Geometry check sheet. Reference: the model listing, model coordinates, mm. A direction names the side the tool comes from. Coordinates: 2 decimals unless noted, no trailing zeros. Order: outer loops, then holes, each group sorted by start corner. A loop starts at its lowest first (then second) coordinate and runs counter-clockwise, first axis right, second up.
Autodesk Inventor part; units mm, degrees
ref_plane "YZ Plane" through (0, 0, 0) normal (1, 0, 0) x (0, 1, 0)
ref_plane "XZ Plane" through (0, 0, 0) normal (0, 1, 0) x (-1, 0, 0)
ref_plane "XY Plane" through (0, 0, 0) normal (0, 0, 1) x (1, 0, 0)
sketch "Эскиз1" plane through (0, 0, 0) normal (0, 1, 0) x (-1, 0, 0)
  line L0 (0, 0) -> (22, 0)
  line L1 (22, 0) -> (22, -27)
  line L2 (22, -27) -> (0, -27)
  line L3 (0, -27) -> (0, 0)
  dimension "d0" = 22
  dimension "d1" = 27
extrude "Выдавливание1" add sketch "Эскиз1" along normal blind 1.4
sketch "Эскиз2" plane through (0, 0, 0) normal (0, -1, 0) x (1, 0, 0)
  circle A0 centre (-5.75, -4.75) radius 3.9
  circle A1 centre (-5.75, -22.25) radius 3.9
  line L0 (-22, 0) -> (0, 0)
  line L1 (0, 0) -> (0, -27)
  line L2 (0, -27) -> (-22, -27)
  dimension "d4" = 7.8
  dimension "d5" = 7.8
  dimension "d6" = 4.75
  dimension "d7" = 5.75
  dimension "d8" = 5.75
  dimension "d9" = 4.75
extrude "Выдавливание2" add sketch "Эскиз2" along normal blind 11.5
sketch "Эскиз3" plane through (-5.75, -11.5, -22.25) normal (0, -1, 0) x (1, 0, 0)
  circle A0 centre (0, 0) radius 2.75
  point P0 (5.75, 22.25)
  dimension "d12" = 5.5
extrude "Выдавливание3" cut sketch "Эскиз3" against normal blind 3
sketch "Эскиз4" plane through (-5.75, -11.5, -4.75) normal (0, -1, 0) x (1, 0, 0)
  circle A0 centre (0, 0) radius 2.75
  point P0 (5.75, 4.75)
  dimension "d13" = 5.5
extrude "Выдавливание4" cut sketch "Эскиз4" against normal blind 3
sketch "Эскиз5" plane through (0, 1.4, 0) normal (0, 1, 0) x (1, 0, 0)
  circle A0 centre (-5.75, 4.75) radius 3.9
  circle A1 centre (-5.75, 4.75) radius 1.75
  circle A2 centre (-5.75, 22.2717) radius 1.75
  point P0 (0, 0)
  dimension "d20" = 3.5
  dimension "d21" = 3.5
extrude "Выдавливание5" cut sketch "Эскиз5" against normal blind 11.5 contours A1 | A2
sketch "Эскиз6" plane through (0, 1.4, 0) normal (0, 1, 0) x (1, 0, 0)
  circle A0 centre (-5.75, 4.75) radius 2.75
  circle A1 centre (-5.75, 4.75) radius 3.125
  circle A2 centre (-5.75, 22.25) radius 2.75
  circle A3 centre (-5.75, 22.25) radius 3.125
  point P0 (0, 0)
  dimension "d24" = 6.25
  dimension "d25" = 6.25
extrude "Выдавливание6" cut sketch "Эскиз6" against normal blind 6.3 contours A0 | A1 | A2 | A3
properties part number "Крышка для клеммы"
Item 1: Sectioned sample at D-D (z = -24.5). Record the cut outline in (x, y), and give its area (3 significant figures).
Item 2: Sectioned sample at B-B (y = -4.25). Record the cut outline in (x, z) (3 decimals).
Item 3: Release check for a two-part mould opening along Z. For faces 1 (the face through (-8.23, -1.71, -2.85)), 2 (the face through (-3, -11.5, -24)), 3 (the face through (-11, 1, 0)), 4 (the face through (-11, 1, -27)) record: pulls with the +Z half, pulls with the -Z half, needs draft (parallel to the pull), parting line crosses it, or undercut.
Item 4: Tool access check on faces 5 (the face through (-4, -4.9, -3)), 6 (the face through (-3.95, -5.67, -18.79)), 7 (the face through (-7, -11.5, -2)). Record the directions out of +Z, -Z, +X, -X, +Y, -Y that give a thin tool (end or side, any length) a straight path to the whole face; none if there is none.
Item 5: Thickness scan on line 1 along Z through (x, y) = (-5.75, -9.55); line 2 along Z through (x, y) = (-5.75, -5.75); line 3 along Y through (x, z) = (-16.75, -6.5). Record the ranges inside material, lowest first.
Item 6: Depth check by flat-ended pin: P1, Ø6, axis at x = -7.5, z = -11.5, coming from the -Y side; P2, Ø4, axis at y = -4.5, z = -23.5, coming from the -X side; P3, Ø1.9, axis at x = -6, z = -23.5, coming from the +Y side. Enter the tip coordinate at first touch or a pass-through.
Item 7: Sectioned sample at C-C (x = -5.75). Give the number of separate pieces and of enclosed holes in the cut face, and give its area (4 significant figures).
Item 8: Sectioned sample at A-A (z = -4.75). Record the cut outline in (x, y) (3 decimals), and give its area (3 significant figures).
Geometry check:
1. outline: (-22, 0) - (-8.94, 0) - (-8.94, -11.5) - (-7.33, -11.5) - (-7.33, -8.5) - (-4.17, -8.5) - (-4.17, -11.5) - (-2.56, -11.5) - (-2.56, 0) - (0, 0) - (0, 1.4) - (-3.58, 1.4) - (-3.58, -4.9) - (-7.92, -4.9) - (-7.92, 1.4) - (-22, 1.4) - close
1. area: 67.3 mm2
2. outline: circle Ø7.8 at (-5.75, -22.25); circle Ø7.8 at (-5.75, -4.75); hole circle Ø6.25 at (-5.75, -22.25); hole circle Ø6.25 at (-5.75, -4.75)
3. face 1: undercut
3. face 2: needs draft
3. face 3: pulls with the +Z half
3. face 4: pulls with the -Z half
4. face 5: +Y
4. face 6: -Y
4. face 7: +Z, -Z, +X, -X, -Y
5. line 1: z = -26.15 to -25, -19.5 to -18.35, -8.65 to -7.5, -2 to -0.85
5. line 2: z = -26.15 to -24.02, -20.52 to -18.35, -8.65 to -6.5, -3 to -0.85
5. line 3: y = 0 to 1.4
6. P1: stops at y = 0
6. P2: stops at x = -9.65
6. P3: stops at y = -4.9
7. separate pieces: 3
7. enclosed holes: 0
7. area: 80.25 mm2
8. outline: (-22, 0) - (-9.65, 0) - (-9.65, -11.5) - (-8.5, -11.5) - (-8.5, -8.5) - (-7.5, -8.5) - (-7.5, -4.9) - (-8.875, -4.9) - (-8.875, 1.4) - (-22, 1.4) - close; (-4, -8.5) - (-3, -8.5) - (-3, -11.5) - (-1.85, -11.5) - (-1.85, 0) - (0, 0) - (0, 1.4) - (-2.625, 1.4) - (-2.625, -4.9) - (-4, -4.9) - close
8. area: 52.0 mm2
